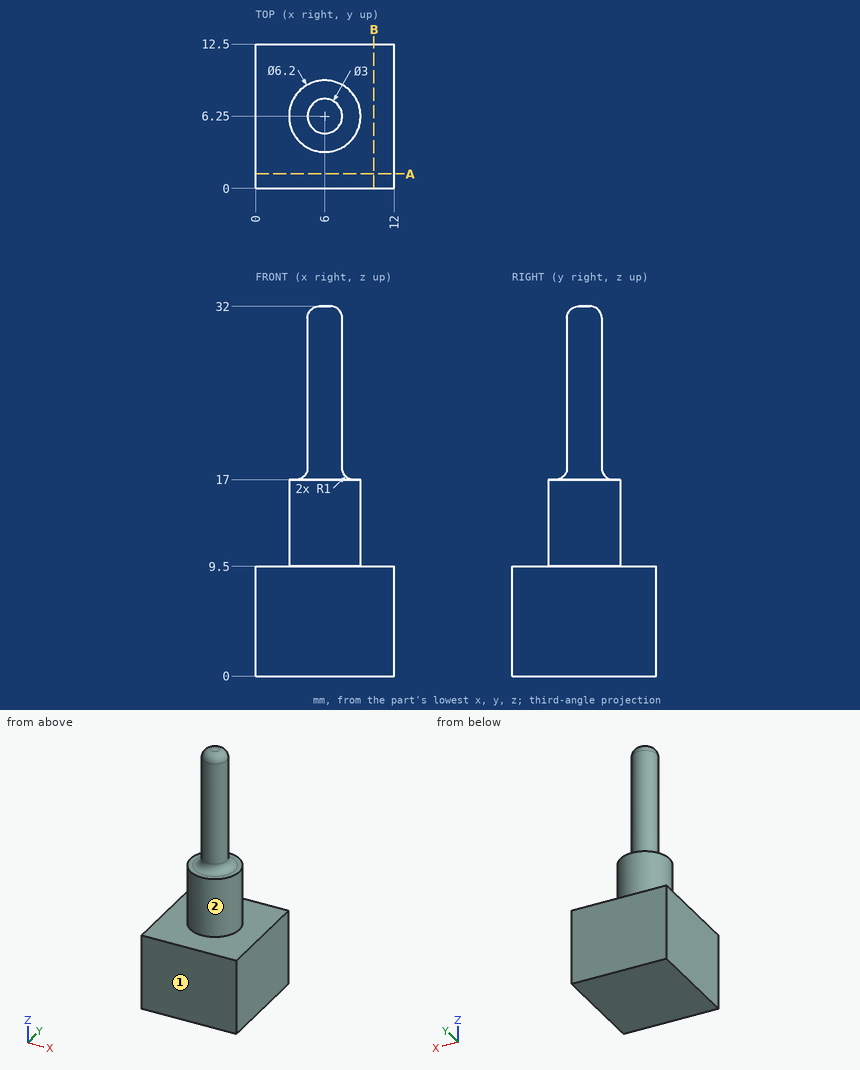
Geometry check sheet. Reference: drawing and pictorial views, mm from the part's lowest x, y, z. A direction names the side the tool comes from. Round coordinates to 2 decimals unless told otherwise and drop trailing zeros. Order: outer loops, then holes, each group sorted by start corner. A loop starts at its lowest first (then second) coordinate and runs counter-clockwise, first axis right, second up. Notation, with made-up numbers: M 47.5,29 L 88.5,29 A31 cw 88.5,54 Z; hole C -22,-35 d6. An arc over 180 degrees is marked long. Answer in a Markdown table with one row per item.
(1) Sectioned sample at B-B, the plane x = 10.25. Record the cut outline in (y, z), and give its area (3 significant figures).
Responses:
| item | result |
|---|---|
| outline | M 0,0 L 12.5,0 L 12.5,9.5 L 0,9.5 Z |
| area | 119 mm² |
(2) Go/stop test with flat-tipped pins: P1, Ø1, axis at x = 6.5, y = 11, coming from the +Z side; P2, Ø3, axis at x = 8.5, z = 23.5, coming from the -Y side; P3, Ø5, axis at y = 3, z = 16, coming from the -X side. Record where each tip stops, or that it passes through.
Responses:
| item | result |
|---|---|
| P1 | stops at z = 9.5 |
| P2 | stops at y = 5.13 |
| P3 | stops at x = 2.99 |
(3) Scan lines: probe 1 along Z at (x, y) = (8.5, 6.75); probe 2 along Z at (x, y) = (10, 1.75); probe 3 along X at (y, z) = (5.5, 30.5). Record each from-to range of solid material in increasing order. Write a range as from..to.
Responses:
| item | result |
|---|---|
| probe 1 | z = 0..17 |
| probe 2 | z = 0..9.5 |
| probe 3 | x = 4.7..7.3 |
(4) Sectioned sample at A-A, the plane y = 1.25. Record the cut outline in (x, z), and give its area (3 significant figures).
Responses:
| item | result |
|---|---|
| outline | M 0,0 L 12,0 L 12,9.5 L 0,9.5 Z |
| area | 114 mm² |
(5) Tool access check on the marked faces 1 and 2. Record the directions out of +Z, -Z, +X, -X, +Y, -Y that give a thin tool (end or side, any length) a straight path to the whole face; none if there is none.
Responses:
| item | result |
|---|---|
| face 1 | +Z, -Z, +X, -X, -Y |
| face 2 | +Z |
